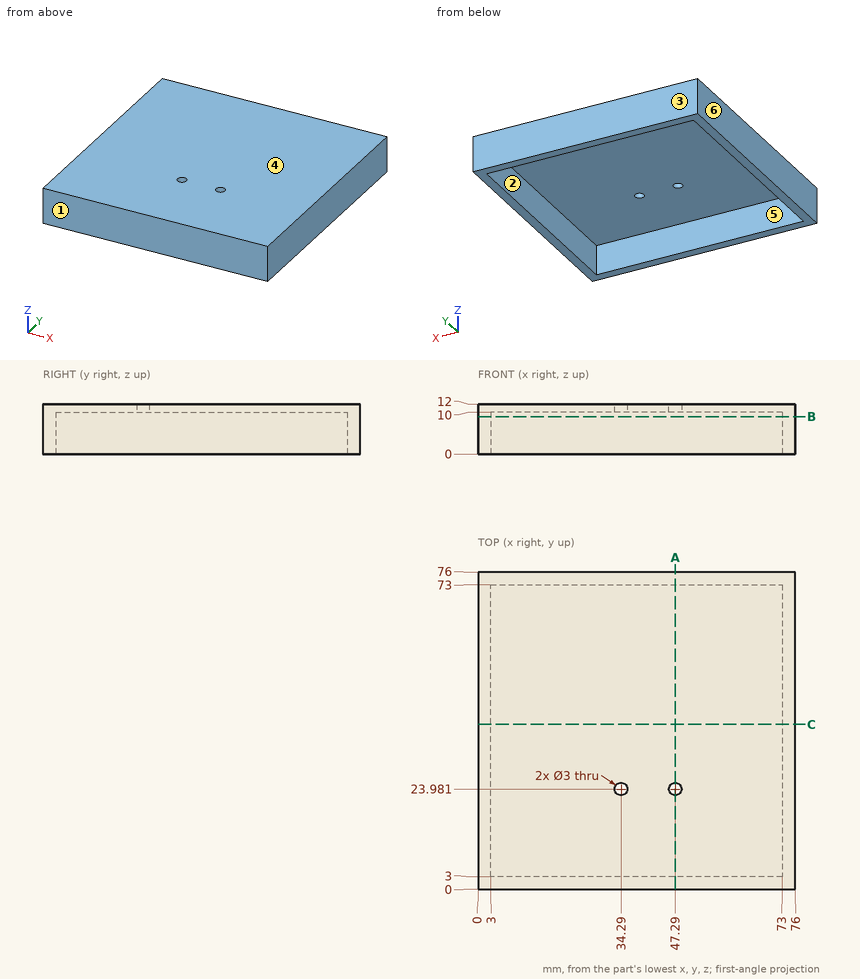
Geometry check sheet. Reference: drawing and pictorial views, mm from the part's lowest x, y, z. A direction names the side the tool comes from. Round coordinates to 2 decimals unless told otherwise and drop trailing zeros. Write each loop counter-clockwise with the first axis right and the second up, starting at its lowest first coordinate (ties: lowest second). Pieces come first, ordered by that corner, then holes.
Item 1: Go/stop test with a flat-tipped pin: pin 1 Ø2 at (x, y) = (39.5, 19.5) entering from -Z. Record where the tip stops, or that it passes through.
Determined:
pin 1: stops at z = 10
Item 2: Access from +Z, -Z, +X, -X, +Y, -Y to the whole of each face (thin tool, end or side, straight path). Record for the marked faces 5 and 6.
Determined:
face 5: -Z
face 6: +Z, -Z, -X, +Y, -Y
Item 3: Section check B-B (z = 9). Record the boundary of the cut face in (x, y).
Determined:
outline: (0, 0) - (76, 0) - (76, 76) - (0, 76) - close; hole (3, 3) - (73, 3) - (73, 73) - (3, 73) - close
Item 4: Section check A-A (x = 47.29). Record the boundary of the cut face in (y, z), plus the area to 3 significant figures.
Determined:
outline: (0, 0) - (3, 0) - (3, 10) - (22.48, 10) - (22.48, 12) - (0, 12) - close; (25.48, 10) - (73, 10) - (73, 0) - (76, 0) - (76, 12) - (25.48, 12) - close
area: 206 mm2
Item 5: Section check C-C (y = 39.5). Record the boundary of the cut face in (x, z).
Determined:
outline: (0, 0) - (3, 0) - (3, 10) - (73, 10) - (73, 0) - (76, 0) - (76, 12) - (0, 12) - close
Item 6: Material ranges on line 1 along X through (y, z) = (16, 2.5); line 2 along Y through (x, z) = (47.29, 10.5), recorded low to high.
Determined:
line 1: x = 0 to 3, 73 to 76
line 2: y = 0 to 22.48, 25.48 to 76
Item 7: Mould release check, pull along Y, two halves, no side actions. Record for the marked faces 1, 2, 3 and 4: +Y half, -Y half, draft (parallel to the pull), parting line (faces both ways), or undercut.
Determined:
face 1: -Y half
face 2: undercut
face 3: +Y half
face 4: draft
